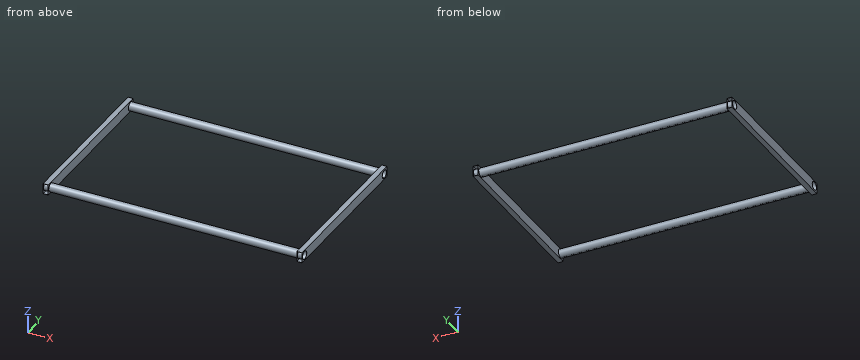
from build123d import *

# Parameters (mm, degrees)
SKETCH3_W             = 50.5
SKETCH3_H             = 101
SKETCH3_W_2           = 48.5
SKETCH3_H_2           = 99
BOSS_EXTRUDE1_DEPTH   = 1600
BOSS_EXTRUDE1_2_DEPTH = 1600
SKETCH4_R             = 39.5
CUT_EXTRUDE1_DEPTH    = 1
SKETCH5_R             = 39.5
CUT_EXTRUDE2_DEPTH    = 1
SKETCH6_R             = 40.5
CUT_EXTRUDE3_DEPTH    = 2401
BOSS_EXTRUDE2_DEPTH   = 2498


with BuildPart() as part:
    # Sketch3 → Boss-Extrude1 (new body)
    with BuildSketch(Plane(origin=(0, 0, 0), x_dir=(1, 0, 0), z_dir=(0, 1, 0))):
        with Locations((-25.25, 0)):
            Rectangle(SKETCH3_W, SKETCH3_H)
        with Locations((-25.25, 0)):
            Rectangle(SKETCH3_W_2, SKETCH3_H_2, mode=Mode.SUBTRACT)
    extrude(amount=BOSS_EXTRUDE1_DEPTH)

    # Sketch5 → Cut-Extrude2 (cut)
    with BuildSketch(Plane.ZY.offset(50.5)):
        with Locations((0, 50)):
            Circle(SKETCH5_R)
        with Locations((0, 1550)):
            Circle(SKETCH5_R)
    extrude(amount=-CUT_EXTRUDE2_DEPTH, mode=Mode.SUBTRACT)


with BuildPart() as body_2:
    # Sketch3 → Boss-Extrude1 2 (new body)
    with BuildSketch(Plane(origin=(0, 0, 0), x_dir=(1, 0, 0), z_dir=(0, 1, 0))):
        with Locations((2424.25, 0)):
            Rectangle(SKETCH3_W, SKETCH3_H)
        with Locations((2424.25, 0)):
            Rectangle(SKETCH3_W_2, SKETCH3_H_2, mode=Mode.SUBTRACT)
    extrude(amount=BOSS_EXTRUDE1_2_DEPTH)

    # Sketch4 → Cut-Extrude1 (cut)
    with BuildSketch(Plane(origin=(2449.5, 0, 0), x_dir=(0, 0, -1), z_dir=(1, 0, 0))):
        with Locations((0, 50)):
            Circle(SKETCH4_R)
        with Locations((0, 1550)):
            Circle(SKETCH4_R)
    extrude(amount=-CUT_EXTRUDE1_DEPTH, mode=Mode.SUBTRACT)


with BuildPart() as cut_extrude3_tool:
    # Sketch6 → Cut-Extrude3 (new body)
    with BuildSketch(Plane(origin=(2400, 0, 0), x_dir=(0, 0, -1), z_dir=(1, 0, 0))):
        with Locations((0, 50)):
            Circle(SKETCH6_R)
        with Locations((0, 1550)):
            Circle(SKETCH6_R)
    extrude(amount=-CUT_EXTRUDE3_DEPTH)


with BuildPart() as part_1:
    add(part.part)

    # Cut-Extrude3: cut by cut_extrude3_tool
    add(cut_extrude3_tool.part, mode=Mode.SUBTRACT)



with BuildPart() as body_2_1:
    add(body_2.part)

    # Cut-Extrude3: cut by cut_extrude3_tool
    add(cut_extrude3_tool.part, mode=Mode.SUBTRACT)


with BuildPart() as part_2:
    add(part_1.part)

    add(body_2_1.part)  # Boss-Extrude2 merges body 2
    # Sketch7 → Boss-Extrude2 (add)
    with BuildSketch(Plane.ZY.offset(-2448.5)):
        with BuildLine():
            Line((-39.496835316, 50.5), (-40.496913463, 50.5))
            ThreePointArc((-40.496913463, 50.5), (40.5, 50), (-40.496913463, 49.5))
            Line((-40.496913463, 49.5), (-39.496835316, 49.5))
            ThreePointArc((-39.496835316, 49.5), (39.5, 50), (-39.496835316, 50.5))
        make_face()
        with BuildLine():
            Line((-40.496913463, 1550.5), (-39.496835316, 1550.5))
            ThreePointArc((-39.496835316, 1550.5), (39.5, 1550), (-39.496835316, 1549.5))
            Line((-39.496835316, 1549.5), (-40.496913463, 1549.5))
            ThreePointArc((-40.496913463, 1549.5), (40.5, 1550), (-40.496913463, 1550.5))
        make_face()
    extrude(amount=BOSS_EXTRUDE2_DEPTH)


solid = part_2.part
The listing builds one solid part. Answer for the finished solid, in the listing's coordinates (mm). Coordinates: 2 decimals unless noted, no trailing zeros. Loops run counter-clockwise (first coordinate to the right, second up) from the corner with the lowest first, then second, coordinate; pieces in that order, holes last. Notation, with made-up numbers: (77, 84) -> (132, 84) arc R10 ccw to (132, 89) -> close; hole circle Ø4 at (88.25, 61). An arc over 180 degrees is marked (long way). Answer in a Markdown table with one row per item. Add a question column.
1. The part is cut by section A-A, the plane y = 1070.5. Write down the section's boundary in (x, z).
2. The part is cut by section B-B, the plane x = 1412. Write down the section's boundary in (y, z).
3. Flat-ended cylindrical pins translate along their axes: P1, Ø3, axis at x = 1198, z = 7, coming from the +Y side; P2, Ø6, axis at x = 2043.5, z = -11.5, coming from the -Y side; P3, Ø6, axis at x = 2086, z = -15, coming from the -Y side. Find the tip coordinate at first contact, or state that the pin passes through.
4. The part is cut by section C-C, the plane z = 0. Count the separate pieces of the cut face and the enclosed holes in it, then the cut area to 3 significant figures.
5. Consider line 1 (X direction, y = 1485.5, z = -35); line 2 (Y direction, x = 2449, z = 0); line 3 (Y direction, x = 1323.5, z = 0). Determine where each line is inside the solid, lowest interval first. Write a range as [from, to].
Answer below:
| question | item | result |
|---|---|---|
| 1 | outline | (-50.5, -50.5) -> (0, -50.5) -> (0, 50.5) -> (-50.5, 50.5) -> close; (2399, -50.5) -> (2449.5, -50.5) -> (2449.5, 50.5) -> (2399, 50.5) -> close; hole (-49.5, -49.5) -> (-1, -49.5) -> (-1, 49.5) -> (-49.5, 49.5) -> close; hole (2400, -49.5) -> (2448.5, -49.5) -> (2448.5, 49.5) -> (2400, 49.5) -> close |
| 2 | outline | (49.5, -40.5) -> (49.5, -39.5) arc R39.5 cw (long way) to (50.5, -39.5) -> (50.5, -40.5) arc R40.5 ccw (long way) to start; (1549.5, -40.5) -> (1549.5, -39.5) arc R39.5 cw (long way) to (1550.5, -39.5) -> (1550.5, -40.5) arc R40.5 ccw (long way) to start |
| 3 | P1 | y = 1590.12 |
| 3 | P2 | y = 10.4 |
| 3 | P3 | y = 11.32 |
| 4 | separate pieces | 3 |
| 4 | enclosed holes | 3 |
| 4 | area | 15,800 mm2 |
| 5 | line 1 | [-50.5, -49.5], [-1, 0], [2399, 2400], [2448.5, 2449.5] |
| 5 | line 2 | [0, 10.5], [89.5, 1510.5], [1589.5, 1600] |
| 5 | line 3 | [9.5, 10.5], [89.5, 90.5], [1509.5, 1510.5], [1589.5, 1590.5] |
